from build123d import *

# Parameters (mm, degrees)
F1_DEPTH = 40
F2_DEPTH = 1
F4_DEPTH = 1


with BuildPart() as f1:
    # F0 (on Top) → F1 (new body)
    with BuildSketch(Plane.XY):
        with BuildLine():
            ThreePointArc((-1.5, 7.3484692283), (-4.7434164903, -5.8094750193), (7.5, 0))
            ThreePointArc((7.5, 0), (5.8094750193, 4.7434164903), (1.5, 7.3484692283))
            Line((1.5, 7.3484692283), (1.5, 0))
            ThreePointArc((1.5, 0), (0, -1.5), (-1.5, 0))
            Line((-1.5, 0), (-1.5, 7.3484692283))
        make_face()
        with BuildLine():
            Line((1.5, 0), (1.5, 7.3484692283))
            ThreePointArc((1.5, 7.3484692283), (0, 7.5), (-1.5, 7.3484692283))
            Line((-1.5, 7.3484692283), (-1.5, 0))
            ThreePointArc((-1.5, 0), (0, -1.5), (1.5, 0))
        make_face()
    extrude(amount=F1_DEPTH)

    # F0 (on Top) → F2 (cut)
    with BuildSketch(Plane.XY):
        with BuildLine():
            Line((1.5, 0), (1.5, 7.3484692283))
            ThreePointArc((1.5, 7.3484692283), (0, 7.5), (-1.5, 7.3484692283))
            Line((-1.5, 7.3484692283), (-1.5, 0))
            ThreePointArc((-1.5, 0), (0, -1.5), (1.5, 0))
        make_face()
    extrude(amount=F2_DEPTH, mode=Mode.SUBTRACT)

    # F3 (on face) → F4 (cut)
    with BuildSketch(Plane.XY.offset(40)):
        with BuildLine():
            ThreePointArc((-1.5, 0), (0, -1.5), (1.5, 0))
            Line((1.5, 0), (1.5, 7.3484692283))
            ThreePointArc((1.5, 7.3484692283), (0, 7.5), (-1.5, 7.3484692283))
            Line((-1.5, 7.3484692283), (-1.5, 0))
        make_face()
    extrude(amount=-F4_DEPTH, mode=Mode.SUBTRACT)


solid = f1.part
Geometry: final body of the model. Coordinates: model frame, mm. A direction names the side the tool comes from. Round coordinates to 2 decimals unless told otherwise and drop trailing zeros. Loops run counter-clockwise (first coordinate to the right, second up) from the corner with the lowest first, then second, coordinate; pieces in that order, holes last. Notation, with made-up numbers: M 53,72.25 L 95,72.25 A20 ccw 95,90.25 Z; hole C -7,4 d7. An arc over 180 degrees is marked long. Put each result on its own line as item: value. Start each with the question number.
(1) Material intervals for line 1 along Y through (x, z) = (0.25, 29); line 2 along X through (y, z) = (5.25, 13), sorted ascending. Write a range as [from, to].
(2) Section query A-A (x = 0). Return loops of the section in (y, z).
(3) Draft query along X for faces 4 (the face through (-1.5, 3.7, 39.5)), 5 (the face through (0, -2, 40)). Return one class per face: +X half, -X half, draft (parallel to the pull), parting line (faces both ways), or undercut.
(4) Section query C-C (z = 9.5). Return loops of the section in (x, y).
(5) Section query D-D (y = -6). Return loops of the section in (x, z), then the cut area to 3 significant figures.
(6) Set-up query: faces 1 (the face through (0, -1.5, 0.5)), 2 (the face through (0, -2, 0)), 3 (the face through (0, 3, 39)). Return all of +Z, -Z, +X, -X, +Y, -Y with unobstructed straight access to the full face (end or side cutting, diameter ignored); none if empty.
(7) Section query B-B (y = 5). Return loops of the section in (x, z), then the cut area to 3 significant figures.
(8) Contact query for flat-ended pins moving along their axis: pin 1 Ø1 at (y, z) = (5.5, 31) entering from +X; pin 2 Ø1.1 at (y, z) = (3.5, 39.5) entering from -X; pin 3 Ø0.8 at (y, z) = (4, 0.5) entering from +X. Output: stop coordinate, or through.
Findings below:
1. line 1: y = [-7.5, 7.5]
1. line 2: x = [-5.36, 5.36]
2. outline: M -7.5,0 L -1.5,0 L -1.5,1 L 7.5,1 L 7.5,39 L -1.5,39 L -1.5,40 L -7.5,40 Z
3. face 4: undercut
3. face 5: draft
4. outline: C 0,0 d15
5. outline: M -4.5,0 L 4.5,0 L 4.5,40 L -4.5,40 Z
5. area: 360 mm2
6. face 1: -Z, +Y
6. face 2: -Z, +X, -X, +Y, -Y
6. face 3: +Z, +Y
7. outline: M -5.59,0 L -1.5,0 L -1.5,1 L 1.5,1 L 1.5,0 L 5.59,0 L 5.59,40 L 1.5,40 L 1.5,39 L -1.5,39 L -1.5,40 L -5.59,40 Z
7. area: 441 mm2
8. pin 1: stops at x = 5.59
8. pin 2: stops at x = -6.9
8. pin 3: stops at x = 6.58
